Can you work these out from the model? Positions are in its coordinate system, mm. Face numbers are marked on the shaded views. A direction names the side the tool comes from. Coordinates: 2 decimals unless noted, no trailing zeros. Order: outer loops, then holes, each group sorted by start corner. A loop starts at its lowest first (then second) coordinate and runs counter-clockwise, first axis right, second up. Notation, with made-up numbers: (63.25, 85.25) -> (70.25, 85.25) arc R12 cw to (70.25, 103.25) -> close; hole circle Ø10 at (41.25, 21.5). An arc over 180 degrees is marked (long way). Answer in a Markdown table with one row per item.
```python
from build123d import *

# Parameters (mm, degrees)
SKETCH1_W           = 11.021234102
SKETCH1_H           = 12.740456306
BOSS_EXTRUDE1_DEPTH = 10
SKETCH2_W           = 2.201611783
SKETCH2_H           = 2.854410055
SKETCH2_W_2         = 3.227403416
SKETCH2_H_2         = 3.863656662
SKETCH2_W_3         = 3.078498179
SKETCH2_H_3         = 3.185310582
SKETCH2_W_4         = 4.766090866
SKETCH2_H_4         = 4.591637821
CUT_EXTRUDE1_DEPTH  = 2
SKETCH3_W           = 4.20243669
SKETCH3_H           = 4.351341928
CUT_EXTRUDE2_DEPTH  = 5


with BuildPart() as part:
    # Sketch1 → Boss-Extrude1 (new body)
    with BuildSketch(Plane(origin=(0, 0, 0), x_dir=(1, 0, 0), z_dir=(0, 1, 0))):
        Rectangle(SKETCH1_W, SKETCH1_H)
    extrude(amount=BOSS_EXTRUDE1_DEPTH)

    # Sketch2 → Cut-Extrude1 (cut)
    with BuildSketch(Plane(origin=(0, 10, 0), x_dir=(1, 0, 0), z_dir=(0, 1, 0))):
        with Locations((-4.40981116, -4.943023125)):
            Rectangle(SKETCH2_W, SKETCH2_H)
        with Locations((3.896915343, -4.438399822)):
            Rectangle(SKETCH2_W_2, SKETCH2_H_2)
        with Locations((-3.971367962, 4.777572862)):
            Rectangle(SKETCH2_W_3, SKETCH2_H_3)
        with Locations((3.127571618, 4.074409242)):
            Rectangle(SKETCH2_W_4, SKETCH2_H_4)
    extrude(amount=-CUT_EXTRUDE1_DEPTH, mode=Mode.SUBTRACT)

    # Sketch3 → Cut-Extrude2 (cut)
    with BuildSketch(Plane.XZ):
        Rectangle(SKETCH3_W, SKETCH3_H)
    extrude(amount=-CUT_EXTRUDE2_DEPTH, mode=Mode.SUBTRACT)


solid = part.part
```
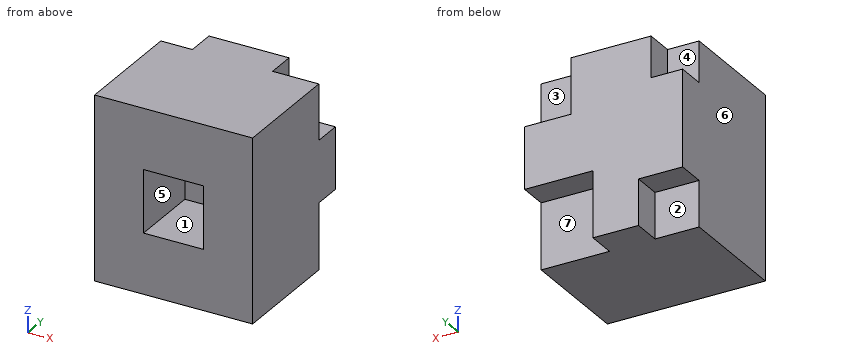
(1) I need wall thicknesses on line 1 (Z direction, x = 1.75, y = 3.25); line 2 (X direction, y = 1, z = -0.5); line 3 (Y direction, x = 1.5, z = -5.5). Which ranges of each line are inside material? Lowest first, please. Write a range as [from, to].
Response values:
| item | result |
|---|---|
| line 1 | [-6.37, -2.18], [2.18, 6.37] |
| line 2 | [-5.51, -2.1], [2.1, 5.51] |
| line 3 | [0, 8] |
(2) Will these pins go through, and if not, where does the flat tip stop? pin 1 Ø0.6 at (y, z) = (9, 5) entering from -X; pin 2 Ø2 at (x, z) = (-1, 0.5) entering from -Y; pin 3 Ø0.6 at (x, y) = (4, 9) entering from -Z.
Response values:
| item | result |
|---|---|
| pin 1 | x = -3.31 |
| pin 2 | y = 5 |
| pin 3 | z = -1.78 |
(3) On a 3-axis mill with a long thin cutter (end or side, diameter ignored), from which of +Z, -Z, +X, -X, +Y, -Y can I reach the whole of each face in a straight line? I mean the marked faces 1, 2, 3 and 4. Say none if no direction works.
Response values:
| item | result |
|---|---|
| face 1 | -Y |
| face 2 | -Z, -X, +Y |
| face 3 | +Z, +X, +Y |
| face 4 | +Z, -X, +Y |
(4) Suppose I cut it at C-C (z = 1.5). Please give me the cut outline in (x, y).
Response values:
| item | result |
|---|---|
| outline | (-5.51, 0) -> (-2.1, 0) -> (-2.1, 5) -> (2.1, 5) -> (2.1, 0) -> (5.51, 0) -> (5.51, 10) -> (-5.51, 10) -> close |
(5) Suppose I cut it at A-A (x = 0.5). Please give me the cut outline in (y, z).
Response values:
| item | result |
|---|---|
| outline | (0, -6.37) -> (10, -6.37) -> (10, 6.37) -> (0, 6.37) -> (0, 2.18) -> (5, 2.18) -> (5, -2.18) -> (0, -2.18) -> close |
(6) We'd pull the mould along X, two halves only. Please class the marked faces 5, 6 and 7: +X half, -X half, draft (parallel to the pull), parting line (faces both ways), or undercut.
Response values:
| item | result |
|---|---|
| face 5 | undercut |
| face 6 | -X half |
| face 7 | draft |
(7) Suppose I cut it at B-B (y = 3.25). Please give me the cut outline in (x, z), and give its area (3 significant figures).
Response values:
| item | result |
|---|---|
| outline | (-5.51, -6.37) -> (5.51, -6.37) -> (5.51, 6.37) -> (-5.51, 6.37) -> close; hole (-2.1, -2.18) -> (2.1, -2.18) -> (2.1, 2.18) -> (-2.1, 2.18) -> close |
| area | 122 mm2 |
(8) Suppose I cut it at D-D (y = 8.5). Please give me the cut outline in (x, z).
Response values:
| item | result |
|---|---|
| outline | (-5.51, -3.18) -> (-2.43, -3.18) -> (-2.43, -6.37) -> (0.74, -6.37) -> (0.74, -1.78) -> (5.51, -1.78) -> (5.51, 2.51) -> (2.28, 2.51) -> (2.28, 6.37) -> (-3.31, 6.37) -> (-3.31, 3.52) -> (-5.51, 3.52) -> close |
